```python
from build123d import *

# Parameters (mm, degrees)
CROQUIS1_R                                           = 1
CROQUIS1_R_2                                         = 11.25
SALIENTE_EXTRUIR1_DEPTH                              = 4
CROQUIS2_R                                           = 1
SALIENTE_EXTRUIR2_DEPTH                              = 10.5
CROQUIS3_R                                           = 3
CROQUIS3_R_2                                         = 1.5
CORTAR_EXTRUIR1_DEPTH                                = 9.75
REFRENTADO_PARA_TORNILLO_TAP_N_CON_CABEZ_D           = 3.4
REFRENTADO_PARA_TORNILLO_TAP_N_CON_CABEZ_CSINK_D     = 6.72
REFRENTADO_PARA_TORNILLO_TAP_N_CON_CABEZ_CSINK_ANGLE = 90
REFRENTADO_PARA_TORNILLO_TAP_N_CON_C_2_D             = 3.4
REFRENTADO_PARA_TORNILLO_TAP_N_CON_C_2_CSINK_D       = 6.72
REFRENTADO_PARA_TORNILLO_TAP_N_CON_C_2_CSINK_ANGLE   = 90


with BuildPart() as part:
    # Croquis1 → Saliente-Extruir1 (new body)
    with BuildSketch(Plane.XY):
        with BuildLine():
            Line((-18, 21), (18, 21))
            ThreePointArc((18, 21), (20.121320344, 20.121320344), (21, 18))
            Line((21, 18), (21, -18))
            ThreePointArc((21, -18), (20.121320344, -20.121320344), (18, -21))
            Line((18, -21), (-18, -21))
            ThreePointArc((-18, -21), (-20.121320344, -20.121320344), (-21, -18))
            Line((-21, -18), (-21, 18))
            ThreePointArc((-21, 18), (-20.121320344, 20.121320344), (-18, 21))
        make_face()
        with Locations((-15.5, 15.5)):
            Circle(CROQUIS1_R, mode=Mode.SUBTRACT)
        with Locations((15.5, 15.5)):
            Circle(CROQUIS1_R, mode=Mode.SUBTRACT)
        with Locations((15.5, -15.5)):
            Circle(CROQUIS1_R, mode=Mode.SUBTRACT)
        with Locations((-15.5, -15.5)):
            Circle(CROQUIS1_R, mode=Mode.SUBTRACT)
        Circle(CROQUIS1_R_2, mode=Mode.SUBTRACT)
    extrude(amount=SALIENTE_EXTRUIR1_DEPTH)

    # Croquis2 → Saliente-Extruir2 (add)
    with BuildSketch(Plane.XY.offset(4)):
        with BuildLine():
            Line((-21, -11.25), (21, -11.25))
            Line((21, -11.25), (21, -18))
            ThreePointArc((21, -18), (20.121320344, -20.121320344), (18, -21))
            Line((18, -21), (-18, -21))
            ThreePointArc((-18, -21), (-20.121320344, -20.121320344), (-21, -18))
            Line((-21, -18), (-21, -11.25))
        make_face()
        with Locations((15.5, -15.5)):
            Circle(CROQUIS2_R, mode=Mode.SUBTRACT)
        with Locations((-15.5, -15.5)):
            Circle(CROQUIS2_R, mode=Mode.SUBTRACT)
    extrude(amount=SALIENTE_EXTRUIR2_DEPTH)

    # Croquis3 → Cortar-Extruir1 (cut)
    with BuildSketch(Plane(origin=(0, -11.25, 0), x_dir=(1, 0, 0), z_dir=(0, 1, 0))):
        with Locations(Location((6, -9.25, 0), (0, 0, 180))):
            Circle(CROQUIS3_R)
        with Locations(Location((-10, -9.25, 0), (0, 0, 180))):
            Circle(CROQUIS3_R_2)
    extrude(amount=-CORTAR_EXTRUIR1_DEPTH, mode=Mode.SUBTRACT)

    # Refrentado para tornillo tap_n con cabez (through all)
    with Locations(Plane.XY.offset(4)):
        with Locations((-15.5, 15.5), (15.5, 15.5)):
            CounterSinkHole(REFRENTADO_PARA_TORNILLO_TAP_N_CON_CABEZ_D / 2, REFRENTADO_PARA_TORNILLO_TAP_N_CON_CABEZ_CSINK_D / 2, counter_sink_angle=REFRENTADO_PARA_TORNILLO_TAP_N_CON_CABEZ_CSINK_ANGLE)

    # Refrentado para tornillo tap_n con c 2 (through all)
    with Locations(Plane.XY.offset(14.5)):
        with Locations((-15.5, -15.5), (15.5, -15.5)):
            CounterSinkHole(REFRENTADO_PARA_TORNILLO_TAP_N_CON_C_2_D / 2, REFRENTADO_PARA_TORNILLO_TAP_N_CON_C_2_CSINK_D / 2, counter_sink_angle=REFRENTADO_PARA_TORNILLO_TAP_N_CON_C_2_CSINK_ANGLE)


solid = part.part
```
Model file for the job. Use its own axes, mm. A direction names the side the tool comes from. Give positions to 0.01 mm unless a question says otherwise; leave off trailing zeros. Write each loop counter-clockwise with the first axis right and the second up, starting at its lowest first coordinate (ties: lowest second). Pieces come first, ordered by that corner, then holes. Notation, with made-up numbers: (-26.5, 88.5) - (24.5, 88.5) arc R22 cw to (24.5, 97.5) - close; hole circle Ø7 at (76, 14.5). An arc over 180 degrees is marked (long way). One line per question, with ' | ' between items. Start each with the question number.
(1) Slice it at A-A on y = -15.5. Write the cut outline in (x, z).
(2) Pin check, flat tips, straight feed: P1, Ø3, axis at x = 3, z = 7, coming from the +Y side; P2, Ø3, axis at x = 3.5, y = 10.5, coming from the +Z side; P3, Ø4.5, axis at x = 15.5, y = -15.5, coming from the +Z side. Stop position of each tip, or through.
(3) Slice it at B-B on x = 15.5. Write the cut outline in (y, z).
(4) 3-axis set-ups, long thin cutter, end or side, ignore diameter. For faces 5 (the face through (0, -11.25, 9)), 6 (the face through (20.1, 20.14, 1.97)): which of +Z, -Z, +X, -X, +Y, -Y reach the whole face in a straight line?
(5) Slice it at C-C on z = 13.5. Write the cut outline in (x, y).
(6) Two-plate mould, pull along Y, no slides. Class faces 1 (the face through (-20.14, 20.1, 1.97)), 2 (the face through (21, -4, 2)), 3 (the face through (5.19, -9.98, 1.97)), 4 (the face through (0, -21, 7)): +Y half, -Y half, draft (parallel to the pull), parting line (faces both ways), or undercut.
(7) Wall check: line 1 along X through (y, z) = (15.5, 1.4); line 2 along X through (y, z) = (-17, 2.5). Give the ranges that are in metal, low to high. Write a range as from..to.
(8) Slice it at D-D on y = 0. Write the cut outline in (x, z), plus the area to 3 significant figures.
Results below:
1) outline: (-21, 0) - (-17.2, 0) - (-17.2, 12.84) - (-18.86, 14.5) - (-21, 14.5) - close; (-13.8, 0) - (13.8, 0) - (13.8, 12.84) - (12.14, 14.5) - (-12.14, 14.5) - (-13.8, 12.84) - close; (17.2, 0) - (21, 0) - (21, 14.5) - (18.86, 14.5) - (17.2, 12.84) - close; hole circle Ø3 at (-10, 9.25); hole circle Ø6 at (6, 9.25)
2) P1: y = -11.25 | P2: z = 4 | P3: z = 13.39
3) outline: (-21, 0) - (-17.2, 0) - (-17.2, 12.84) - (-18.86, 14.5) - (-21, 14.5) - close; (-13.8, 0) - (13.8, 0) - (13.8, 2.34) - (12.14, 4) - (-11.25, 4) - (-11.25, 14.5) - (-12.14, 14.5) - (-13.8, 12.84) - close; (17.2, 0) - (21, 0) - (21, 4) - (18.86, 4) - (17.2, 2.34) - close
4) face 5: +Z, +X, -X, +Y | face 6: +Z, -Z, +X, +Y
5) outline: (-21, -18) arc R3 ccw to (-18, -21) - (18, -21) arc R3 ccw to (21, -18) - (21, -11.25) - (-21, -11.25) - close; hole circle Ø4.72 at (-15.5, -15.5); hole circle Ø4.72 at (15.5, -15.5)
6) face 1: +Y half | face 2: draft | face 3: undercut | face 4: -Y half
7) line 1: -21..-17.2, -13.8..13.8, 17.2..21 | line 2: -21..-16.3, -14.7..14.7, 16.3..21
8) outline: (-21, 0) - (-11.25, 0) - (-11.25, 4) - (-21, 4) - close; (11.25, 0) - (21, 0) - (21, 4) - (11.25, 4) - close | area: 78.0 mm^2
